Here's the drawing with two shaded views (mm, measured from the low corner). I have some questions. Round coordinates to 2 decimals unless told otherwise and drop trailing zeros. Write each loop counter-clockwise with the first axis right and the second up, starting at its lowest first coordinate (ties: lowest second). Pieces come first, ordered by that corner, then holes. Notation, with made-up numbers: M 34,-38.75 L 64,-38.75 A18 cw 64,-15.75 Z; hole C -23.75,-37 d11. An arc over 180 degrees is marked long. Use one line per item in the form item = value. Start each with the question number.
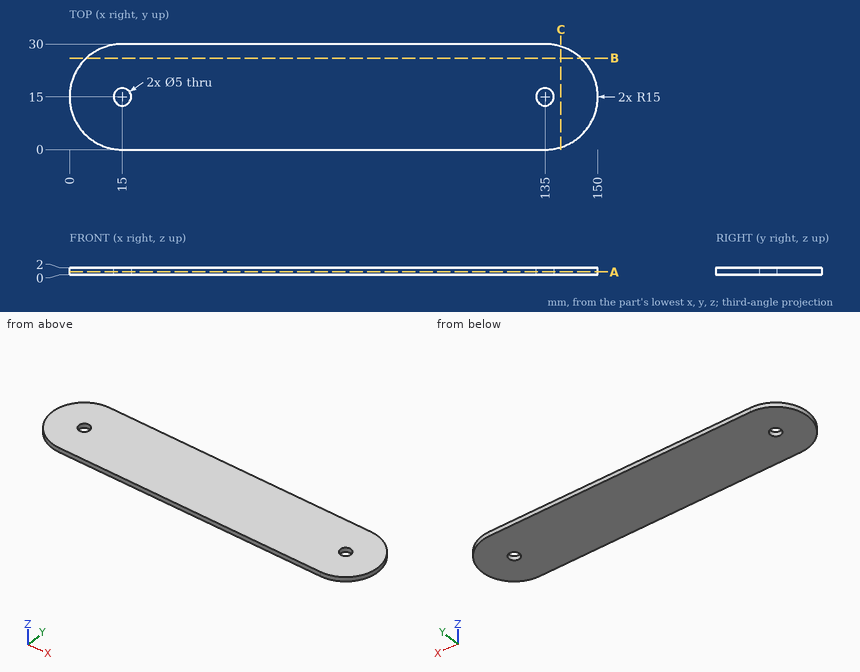
1. If we section it at B-B (y = 26): List the corners of the cut face in (x, z) for me, and give its area (3 significant figures).
2. If we section it at C-C (x = 139.5): List the corners of the cut face in (y, z) for me, and give its area (3 significant figures).
3. If we section it at A-A (z = 0.8): List the corners of the cut face in (x, y) for me, and give its area (3 significant figures).
4. Please list where these lines run through material, in increasing order: line 1 along Y through (x, z) = (135, 0.5); line 2 along X through (y, z) = (15.5, 1.7); line 3 along Y through (x, z) = (135.5, 0.75).
Model answer:
q1.outline = M 4.8,0 L 145.2,0 L 145.2,2 L 4.8,2 Z
q1.area = 281 mm2
q2.outline = M 0.69,0 L 29.31,0 L 29.31,2 L 0.69,2 Z
q2.area = 57.2 mm2
q3.outline = M 15,0 L 135,0 A15 ccw 135,30 L 15,30 A15 ccw Z; hole C 15,15 d5; hole C 135,15 d5
q3.area = 4,270 mm2
q4.line_1 = 0 to 12.5, 17.5 to 30
q4.line_2 = 0.01 to 12.55, 17.45 to 132.55, 137.45 to 149.99
q4.line_3 = 0.01 to 12.55, 17.45 to 29.99
